Geometry check sheet. Reference: drawing and pictorial views, mm from the part's lowest x, y, z. A direction names the side the tool comes from. Coordinates: 2 decimals unless noted, no trailing zeros. Loops run counter-clockwise (first coordinate to the right, second up) from the corner with the lowest first, then second, coordinate; pieces in that order, holes last. Notation, with made-up numbers: M 47,68 L 82,68 A14 ccw 82,74 Z; hole C -4,10.5 d7. An arc over 180 degrees is marked long. Write each question's results on one line, items separated by ' | '. Start each with the question number.
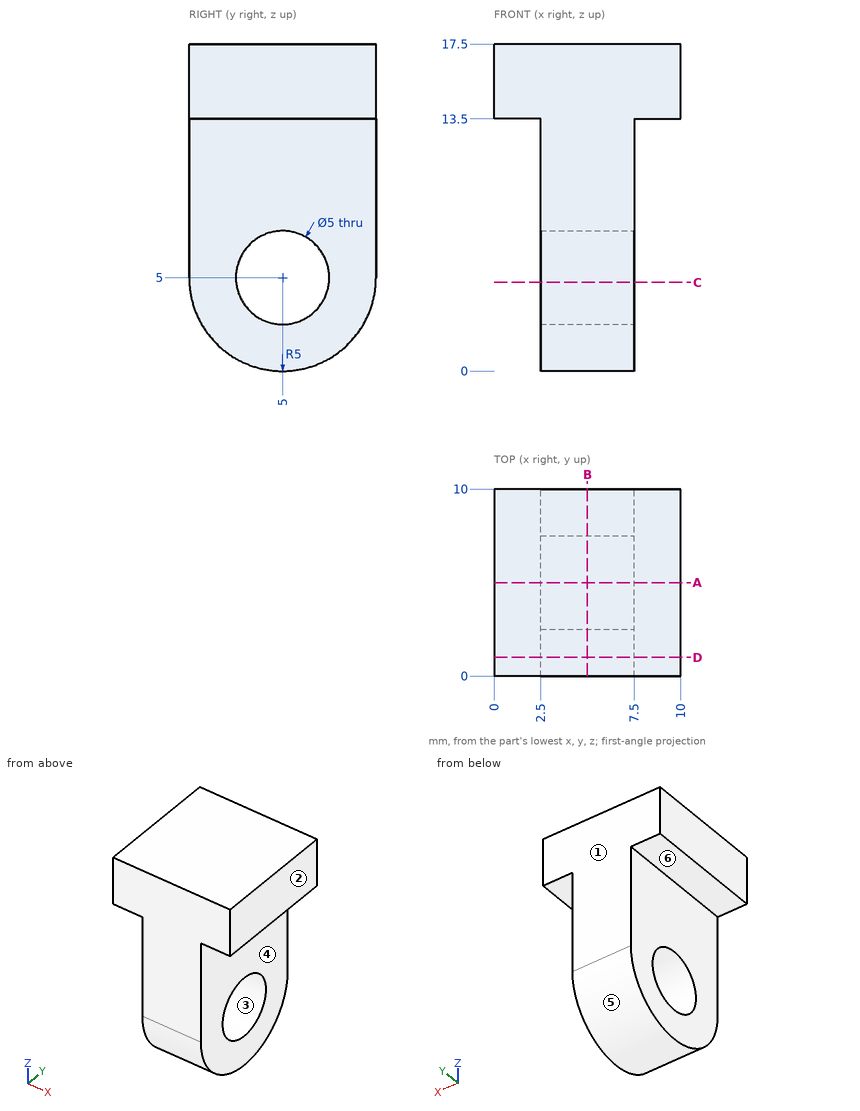
1) Section check D-D (y = 1). Enter the section's corners in (x, z), then the cut area to 3 significant figures.
2) Release check for a two-part mould opening along Y. For the marked faces 1, 2 and 3 record: +Y half, -Y half, draft (parallel to the pull), parting line (faces both ways), or undercut.
3) Thickness scan on probe 1 along Z at (x, y) = (5.8, 5); probe 2 along X at (y, z) = (0.5, 9.75); probe 3 along Z at (x, y) = (7, 7). Record the ranges inside material, lowest first.
4) Section check B-B (x = 5). Enter the section's corners in (y, z), then the cut area to 3 significant figures.
5) Gauge pin test, flat ends, axial feed: P1, Ø2, axis at x = 1, y = 6.5, coming from the -Z side; P2, Ø5, axis at y = 6.5, z = 5, coming from the -X side. Record the tip position at first contact, or that the pin passes through.
6) Section check A-A (y = 5). Enter the section's corners in (x, z), then the cut area to 3 significant figures.
7) Section check C-C (z = 4.75). Enter the section's corners in (x, y), then the cut area to 3 significant figures.
8) Set-up check for the marked faces 4, 5 and 6: record each of +Z, -Z, +X, -X, +Y, -Y from which the full face is reachable in a straight line by a thin tool's end or side.
Return value:
1) outline: M 0,13.5 L 2.5,13.5 L 2.5,2 L 7.5,2 L 7.5,13.5 L 10,13.5 L 10,17.5 L 0,17.5 Z | area: 97.5 mm2
2) face 1: +Y half | face 2: draft | face 3: undercut
3) probe 1: z = 0 to 2.5, 7.5 to 17.5 | probe 2: x = 2.5 to 7.5 | probe 3: z = 0.42 to 3.5, 6.5 to 17.5
4) outline: M 0,5 A5 ccw 10,5 L 10,17.5 L 0,17.5 Z; hole C 5,5 d5 | area: 145 mm2
5) P1: stops at z = 13.5 | P2: stops at x = 2.5
6) outline: M 0,13.5 L 2.5,13.5 L 2.5,7.5 L 7.5,7.5 L 7.5,13.5 L 10,13.5 L 10,17.5 L 0,17.5 Z; M 2.5,0 L 7.5,0 L 7.5,2.5 L 2.5,2.5 Z | area: 82.5 mm2
7) outline: M 2.5,0.01 L 7.5,0.01 L 7.5,2.51 L 2.5,2.51 Z; M 2.5,7.49 L 7.5,7.49 L 7.5,9.99 L 2.5,9.99 Z | area: 25.1 mm2
8) face 4: -Z, +X, +Y, -Y | face 5: -Z, +X, -X | face 6: -Z, -X, +Y, -Y
